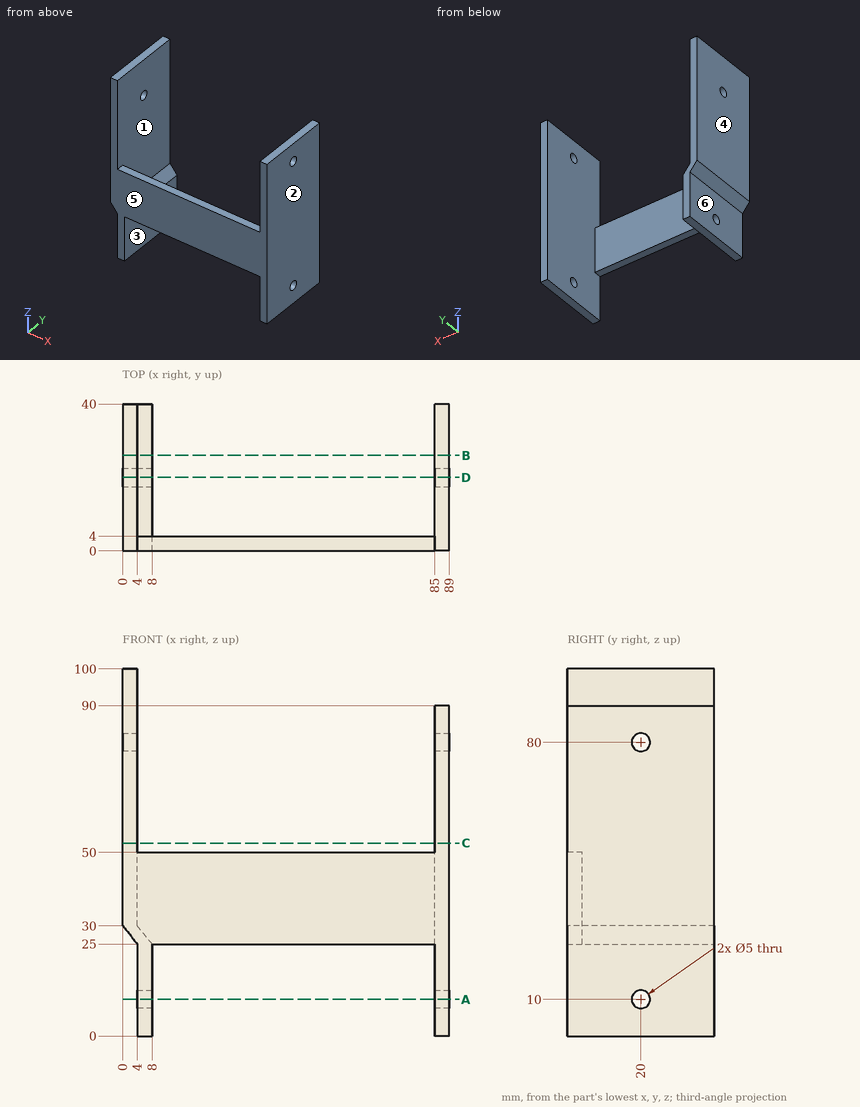
Job drawing, mm, ordinate dimensions from the low corner. One solid piece. A direction names the side the tool comes from. Give positions to 0.01 mm unless a question says otherwise; leave off trailing zeros. Write each loop counter-clockwise with the first axis right and the second up, starting at its lowest first coordinate (ties: lowest second). Pieces come first, ordered by that corner, then holes. Notation, with made-up numbers: M -31,86 L -9,86 A8 ccw -9,90 Z; hole C 18,-30 d1. An arc over 180 degrees is marked long. One line per item, written item: value. Start each with the question number.
Q1. Saw through at B-B, the plane y = 26. Write the cut outline in (x, z).
Q2. Saw through at C-C, the plane z = 52.5. Write the cut outline in (x, y), plus the area to 3 significant figures.
Q3. Drop flat-ended pins along their axis: pin 1 Ø1 at (x, z) = (77.5, 51.5) entering from -Y; pin 2 Ø8 at (x, z) = (53.5, 25) entering from +Y; pin 3 Ø12.5 at (y, z) = (23.5, 13.5) entering from -X; pin 4 Ø12 at (x, y) = (11, 12) entering from +Z. Give the stop position or say it passes through.
Q4. Probe probe 1 along X at (y, z) = (36, 58); probe 2 along X at (y, z) = (25.5, 6.5); probe 3 along Y at (x, z) = (2.85, 80). List the from-to ranges inside material, lowest first. Write a range as [from, to].
Q5. Two-plate mould, pull along X, no slides. Class the marked faces 1, 2, 3 and 4: +X half, -X half, draft (parallel to the pull), parting line (faces both ways), or undercut.
Q6. 3-axis set-ups, long thin cutter, end or side, ignore diameter. For the marked faces 5 and 6: which of +Z, -Z, +X, -X, +Y, -Y reach the whole face in a straight line?
Q7. Saw through at D-D, the plane y = 20. Write the cut outline in (x, z), plus the area to 3 significant figures.
Q8. Saw through at A-A, the plane z = 10. Write the cut outline in (x, y), plus the area to 3 significant figures.
Output values:
1. outline: M 0,30 L 4,25 L 4,0 L 8,0 L 8,25 L 4,30 L 4,100 L 0,100 Z; M 85,0 L 89,0 L 89,90 L 85,90 Z
2. outline: M 0,0 L 4,0 L 4,40 L 0,40 Z; M 85,0 L 89,0 L 89,40 L 85,40 Z
2. area: 320 mm²
3. pin 1: passes through
3. pin 2: stops at y = 4
3. pin 3: stops at x = 4
3. pin 4: stops at z = 28.75
4. probe 1: x = [0, 4], [85, 89]
4. probe 2: x = [4, 8], [85, 89]
4. probe 3: y = [0, 17.5], [22.5, 40]
5. face 1: undercut
5. face 2: +X half
5. face 3: undercut
5. face 4: -X half
6. face 5: +Z, -Z, +X, -X, -Y
6. face 6: -Z, -X, +Y, -Y
7. outline: M 0,30 L 4,25 L 4,12.5 L 8,12.5 L 8,25 L 4,30 L 4,77.5 L 0,77.5 Z; M 0,82.5 L 4,82.5 L 4,100 L 0,100 Z; M 4,0 L 8,0 L 8,7.5 L 4,7.5 Z; M 85,0 L 89,0 L 89,7.5 L 85,7.5 Z; M 85,12.5 L 89,12.5 L 89,77.5 L 85,77.5 Z; M 85,82.5 L 89,82.5 L 89,90 L 85,90 Z
7. area: 680 mm²
8. outline: M 4,0 L 8,0 L 8,17.5 L 4,17.5 Z; M 4,22.5 L 8,22.5 L 8,40 L 4,40 Z; M 85,0 L 89,0 L 89,17.5 L 85,17.5 Z; M 85,22.5 L 89,22.5 L 89,40 L 85,40 Z
8. area: 280 mm²
